Part model, mm, in its own coordinate system. A direction names the side the tool comes from. Give positions to 0.01 mm unless a question says otherwise; leave off trailing zeros. Write each loop counter-clockwise with the first axis right and the second up, starting at its lowest first coordinate (ties: lowest second). Pieces come first, ordered by that corner, then holes. Notation, with made-up numbers: M -11.75,-1.75 L 25.25,-1.75 A19 ccw 25.25,25.25 Z; hole C 12.5,75.5 d10. An arc over 180 degrees is marked long. Answer as CSV lines item,"result". Start each with the question number.
1) Slice it at C-C, the plane x = 102. Give the cut face in (y, z), plus the area to 3 significant figures.
2) Wall check: line 1 along Y through (x, z) = (129, 1.45); line 2 along Y through (x, z) = (-22.5, 3.45); line 3 along Y through (x, z) = (-67, 3.1). Give the ranges that are in metal, low to high. Write a range as from..to.
3) Slice it at B-B, the plane x = 32.5. Give the cut face in (y, z).
4) Slice it at A-A, the plane y = -21.5. Give the cut face in (x, z), plus the area to 3 significant figures.
5) Mould opens along Y. For faces 3 (the flat face through (-2, 54.5, 2)), 4 (the cylindrical face through (-125.289, 47.696, 0.493)), 5 (the flat face through (-2, 1, 5)) say: pulls with the +Y half, pulls with the -Y half, needs draft (parallel to the pull), parting line crosses it, or undercut.
6) Pin check, flat tip, straight feed: pin 1 Ø1.5 at (x, y) = (-89.5, -21) entering from -Z. Stop position of the tip, or through.
7) Tool access for faces 1 (the flat face through (-132, -1, 2)), 2 (the flat face through (8.934, -1.638, 1.972)): list every direction of +Z, -Z, +X, -X, +Y, -Y with a clear straight run to the whole face (end or side of a thin tool).
```python
from build123d import *

# Parameters (mm, degrees)
SKETCH1_W                 = 264
SKETCH1_H                 = 109
BOSS_EXTRUDE1_DEPTH       = 5
CUT_EXTRUDE1_DEPTH        = 1
CUT_EXTRUDE2_DEPTH        = 4
FILLET1_R                 = 3
F_3_0MM_DOWEL_HOLE1_D     = 3
F_3_0MM_DOWEL_HOLE1_DEPTH = 15
F_3_0MM_DOWEL_HOLE1_TIP   = 0.901290929


with BuildPart() as part:
    # Sketch1 → Boss-Extrude1 (new body)
    with BuildSketch(Plane.XY):
        Rectangle(SKETCH1_W, SKETCH1_H)
    extrude(amount=BOSS_EXTRUDE1_DEPTH)

    # Sketch2 → Cut-Extrude1 (cut)
    with BuildSketch(Plane(origin=(0, 0, 0), x_dir=(-1, 0, 0), z_dir=(0, 0, -1))):
        with BuildLine():
            Line((121, 49.5), (-121, 49.5))
            ThreePointArc((-121, 49.5), (-125.242640687, 47.742640687), (-127, 43.5))
            Line((-127, 43.5), (-127, -43.5))
            ThreePointArc((-127, -43.5), (-125.242640687, -47.742640687), (-121, -49.5))
            Line((-121, -49.5), (121, -49.5))
            ThreePointArc((121, -49.5), (125.242640687, -47.742640687), (127, -43.5))
            Line((127, -43.5), (127, 43.5))
            ThreePointArc((127, 43.5), (125.242640687, 47.742640687), (121, 49.5))
        make_face()
        with BuildLine():
            Line((121, 47.5), (-121, 47.5))
            ThreePointArc((-121, 47.5), (-123.828427125, 46.328427125), (-125, 43.5))
            Line((-125, 43.5), (-125, -43.5))
            ThreePointArc((-125, -43.5), (-123.828427125, -46.328427125), (-121, -47.5))
            Line((-121, -47.5), (121, -47.5))
            ThreePointArc((121, -47.5), (123.828427125, -46.328427125), (125, -43.5))
            Line((125, -43.5), (125, 43.5))
            ThreePointArc((125, 43.5), (123.828427125, 46.328427125), (121, 47.5))
        make_face(mode=Mode.SUBTRACT)
    extrude(amount=-CUT_EXTRUDE1_DEPTH, mode=Mode.SUBTRACT)

    # Sketch3 → Cut-Extrude2 (cut)
    with BuildSketch(Plane(origin=(0, 0, 0), x_dir=(-1, 0, 0), z_dir=(0, 0, -1))):
        Polygon((-117, 39.5), (-117, -37.249488302), (115.898875272, 39.5), align=None)
        Polygon((-91.878678072, -39.5), (117, 29.333873245), (117, -39.5), align=None)
    extrude(amount=-CUT_EXTRUDE2_DEPTH, mode=Mode.SUBTRACT)

    # Fillet1
    fillet1_edges = [part.edges().sort_by_distance(p)[0] for p in [
        (117, 39.5, 2),
        (-115.898875272, 39.5, 2),
        (117, -37.249488302, 2),
        (-117, -39.5, 2),
        (91.878678072, -39.5, 2),
        (-117, 29.333873245, 2),
    ]]
    fillet(fillet1_edges, radius=FILLET1_R)

    # Ø3.0mm Dowel Hole1
    with Locations(Plane(origin=(0, 0, 0), x_dir=(-1, 0, 0), z_dir=(0, 0, -1))):
        with Locations((-129, -51.5), (-129, 51.5), (129, 51.5), (129, -51.5), (-39, -51.5), (39, -51.5), (39, 51.5), (-39, 51.5), (129, 0), (-129, 0)):
            Hole(F_3_0MM_DOWEL_HOLE1_D / 2, depth=F_3_0MM_DOWEL_HOLE1_DEPTH)
            with Locations((0, 0, -(F_3_0MM_DOWEL_HOLE1_DEPTH + F_3_0MM_DOWEL_HOLE1_TIP / 2))):  # 118° drill point
                Cone(0, F_3_0MM_DOWEL_HOLE1_D / 2, F_3_0MM_DOWEL_HOLE1_TIP, mode=Mode.SUBTRACT)


solid = part.part
```
Found:
1,outline,"M -54.5,0 L -49.5,0 L -49.5,1 L -47.5,1 L -47.5,0 L -32.31,0 L -32.31,4 L 39.5,4 L 39.5,0 L 47.5,0 L 47.5,1 L 49.5,1 L 49.5,0 L 54.5,0 L 54.5,5 L -54.5,5 Z"
1,area,"254 mm²"
2,line 1,"-54.5..-53, -50..-1.5, 1.5..50, 53..54.5"
2,line 2,"-54.5..-39.5, -1.81..8.72, 39.5..54.5"
2,line 3,"-54.5..-39.5, 12.86..23.39, 39.5..54.5"
3,outline,"M -54.5,0 L -49.5,0 L -49.5,1 L -47.5,1 L -47.5,0 L -39.5,0 L -39.5,4 L -19.93,4 L -19.93,0 L -9.4,0 L -9.4,4 L 39.5,4 L 39.5,0 L 47.5,0 L 47.5,1 L 49.5,1 L 49.5,0 L 54.5,0 L 54.5,5 L -54.5,5 Z"
4,outline,"M -132,0 L -127,0 L -127,1 L -125,1 L -125,0 L -117,0 L -117,4 L 37.26,4 L 37.26,0 L 69.21,0 L 69.21,4 L 117,4 L 117,0 L 125,0 L 125,1 L 127,1 L 127,0 L 132,0 L 132,5 L -132,5 Z"
4,area,"508 mm²"
5,face 3,"pulls with the +Y half"
5,face 4,"undercut"
5,face 5,"needs draft"
6,pin 1,"z = 4"
7,face 1,"+Z, -Z, -X, +Y, -Y"
7,face 2,"-Z"
